from build123d import *

# Parameters (mm, degrees)
SZKIC1_R                         = 75
DODANIE_WYCI_GNI_CIE1_DEPTH      = 70
SKORUPA1_T                       = -2.5
SZKIC3_W                         = 13
SZKIC3_H                         = 21
WYTNIJ_WYCI_GNI_CIE1_DEPTH       = 60
SZKIC4_W                         = 9
SZKIC4_H                         = 11
WYTNIJ_WYCI_GNI_CIE2_DEPTH       = 60
DODANIE_WYCI_GNI_CIE2_REACH      = 192.066
DODANIE_WYCI_GNI_CIE2_END_RADIUS = 75
SZKIC7_W                         = 60
SZKIC7_H                         = 35
SZKIC8_W                         = 45.5
SZKIC8_H                         = 26.5
WYTNIJ_WYCI_GNI_CIE4_DEPTH       = 30
ZAOKR_GLENIE1_R                  = 5
WYTNIJ_WYCI_GNI_CIE5_DEPTH       = 14
SZKIC10_R                        = 1.5
WYTNIJ_WYCI_GNI_CIE6_DEPTH       = 10
SZYK_KO_OWY1_COUNT               = 4
PRZECI_CIE1_START                = -75.0000001
PRZECI_CIE1_OUTLINE_W            = 152
PRZECI_CIE1_OUTLINE_H            = 70
PRZECI_CIE1_OUTLINE_W_2          = 13
PRZECI_CIE1_OUTLINE_H_2          = 21
PRZECI_CIE1_OUTLINE_W_3          = 9
PRZECI_CIE1_OUTLINE_H_3          = 11
PRZECI_CIE1_DEPTH                = 75.0000001
SZKIC11_W                        = 10
SZKIC11_H                        = 10
SZKIC11_R                        = 2.5
DODANIE_WYCI_GNI_CIE3_DEPTH      = 4


# Read off the part's stored shape, not the designer's step: Przecięcie1
with BuildPart() as part:
    # Szkic1 → Dodanie-wyciągnięcie1 (new body)
    with BuildSketch(Plane.XY):
        Circle(SZKIC1_R)
    extrude(amount=DODANIE_WYCI_GNI_CIE1_DEPTH)

    # Skorupa1
    skorupa1_openings = [part.faces().sort_by_distance(p)[0] for p in [
        (0, 0, 70),
    ]]
    offset(amount=SKORUPA1_T, openings=skorupa1_openings, kind=Kind.INTERSECTION)

    # Szkic3 → Wytnij-wyciągnięcie1 (cut)
    with BuildSketch(Plane(origin=(0, -75, 0), x_dir=(-1, 0, 0), z_dir=(0, -1, 0))):
        with Locations((0, -35)):
            Rectangle(SZKIC3_W, SZKIC3_H)
    extrude(amount=-WYTNIJ_WYCI_GNI_CIE1_DEPTH, mode=Mode.SUBTRACT)

    # Szkic4 → Wytnij-wyciągnięcie2 (cut)
    with BuildSketch(Plane(origin=(0, -75, 0), x_dir=(-1, 0, 0), z_dir=(0, -1, 0))):
        with Locations((0, -14)):
            Rectangle(SZKIC4_W, SZKIC4_H)
    extrude(amount=-WYTNIJ_WYCI_GNI_CIE2_DEPTH, mode=Mode.SUBTRACT)

    # Dodanie-wyciągnięcie2: up to this cylinder (the profile starts outside it)
    dodanie_wyci_gni_cie2_end = Plane(origin=(0, 0, 35.532003), z_dir=(0, 0, -1)) * Cylinder(DODANIE_WYCI_GNI_CIE2_END_RADIUS, 535.132, mode=Mode.PRIVATE)
    # Szkic7 → Dodanie-wyciągnięcie2 (add, up to the surface)
    with BuildSketch(Plane(origin=(0, 85, 0), x_dir=(-1, 0, 0), z_dir=(0, -1, 0)), mode=Mode.PRIVATE) as dodanie_wyci_gni_cie2_sk1:
        with Locations((0, -35.532003496)):
            Rectangle(SZKIC7_W, SZKIC7_H)
    dodanie_wyci_gni_cie2_tool1 = extrude(dodanie_wyci_gni_cie2_sk1.sketch, amount=DODANIE_WYCI_GNI_CIE2_REACH, mode=Mode.PRIVATE) - dodanie_wyci_gni_cie2_end
    add(dodanie_wyci_gni_cie2_tool1.solids().sort_by_distance((0, 85, 35.532003))[0])

    # Szkic8 → Wytnij-wyciągnięcie4 (cut)
    with BuildSketch(Plane(origin=(0, 85, 0), x_dir=(1, 0, 0), z_dir=(0, 1, 0))):
        with Locations((0, -35.532003496)):
            Rectangle(SZKIC8_W, SZKIC8_H)
    extrude(amount=-WYTNIJ_WYCI_GNI_CIE4_DEPTH, mode=Mode.SUBTRACT)

    # Zaokrąglenie1
    zaokr_glenie1_edges = [part.edges().sort_by_distance(p)[0] for p in [
        (-30, 76.869317712, 18.032003496),
        (-30, 76.869317712, 53.032003496),
        (30, 76.869317712, 18.032003496),
        (30, 76.869317712, 53.032003496),
    ]]
    fillet(zaokr_glenie1_edges, radius=ZAOKR_GLENIE1_R)

    # Szkic9 → Wytnij-wyciągnięcie5 (cut)
    with BuildSketch(Plane(origin=(75, 0, 0), x_dir=(0, 0, -1), z_dir=(1, 0, 0))):
        with BuildLine():
            Line((-55, -12.979686846), (-55, 12.020313154))
            ThreePointArc((-55, 12.020313154), (-50, 17.020313154), (-45, 12.020313154))
            Line((-45, 12.020313154), (-45, -12.979686846))
            ThreePointArc((-45, -12.979686846), (-50, -17.979686846), (-55, -12.979686846))
        make_face()
    extrude(amount=-WYTNIJ_WYCI_GNI_CIE5_DEPTH, mode=Mode.SUBTRACT)

    # Szkic10 → Wytnij-wyciągnięcie6 (cut)
    with BuildSketch(Plane(origin=(53.033008589, 53.033008589, 0), x_dir=(0, 0, -1), z_dir=(0.7071067811865512, 0.7071067811865438, 0))):
        with Locations(Location((-66, 0, 0), (0, 0, 90))):
            Circle(SZKIC10_R)
    wytnij_wyci_gni_cie6 = extrude(amount=-WYTNIJ_WYCI_GNI_CIE6_DEPTH, mode=Mode.SUBTRACT)

    # Szyk kołowy1: Wytnij-wyciągnięcie6 ×4 about axis
    szyk_ko_owy1_axis = Axis((0, 0, 70), (0, 0, -1))
    for i in range(1, SZYK_KO_OWY1_COUNT):
        add(wytnij_wyci_gni_cie6.rotate(szyk_ko_owy1_axis, i * 360 / SZYK_KO_OWY1_COUNT), mode=Mode.SUBTRACT)

    # Przecięcie1 outline → Przecięcie1 (cut)
    with BuildSketch(Plane(origin=(0, 0, 0), x_dir=(1, 0, 0), z_dir=(0, 1, 0)).offset(PRZECI_CIE1_START)):
        with Locations((0, -35)):
            Rectangle(PRZECI_CIE1_OUTLINE_W, PRZECI_CIE1_OUTLINE_H)
        with Locations((0, -35)):
            Rectangle(PRZECI_CIE1_OUTLINE_W_2, PRZECI_CIE1_OUTLINE_H_2, mode=Mode.SUBTRACT)
        with Locations((0, -14)):
            Rectangle(PRZECI_CIE1_OUTLINE_W_3, PRZECI_CIE1_OUTLINE_H_3, mode=Mode.SUBTRACT)
    extrude(amount=PRZECI_CIE1_DEPTH, mode=Mode.SUBTRACT)

    # Szkic11 → Dodanie-wyciągnięcie3 (add)
    # profile 1 of 2: a face of its own
    with BuildSketch(Plane(origin=(0, 0, 0), x_dir=(-1, 0, 0), z_dir=(0, -1, 0))):
        with Locations((47.5, -7.5)):
            Rectangle(SZKIC11_W, SZKIC11_H)
        with Locations(Location((47.5, -8.5, 0), (0, 0, 90))):
            Circle(SZKIC11_R, mode=Mode.SUBTRACT)
    # profile 2 of 2: a face of its own
    with BuildSketch(Plane(origin=(0, 0, 0), x_dir=(-1, 0, 0), z_dir=(0, -1, 0))):
        with Locations((-47.5, -7.5)):
            Rectangle(SZKIC11_W, SZKIC11_H)
        with Locations(Location((-47.5, -8.5, 0), (0, 0, 90))):
            Circle(SZKIC11_R, mode=Mode.SUBTRACT)
    extrude(amount=-DODANIE_WYCI_GNI_CIE3_DEPTH)


solid = part.part
The listing builds one solid part. Answer for the finished solid, in the listing's coordinates (mm). A direction names the side the tool comes from. Coordinates: 2 decimals unless noted, no trailing zeros. Write each loop counter-clockwise with the first axis right and the second up, starting at its lowest first coordinate (ties: lowest second). Pieces come first, ordered by that corner, then holes. Notation, with made-up numbers: (65.25, 23) -> (108.25, 23) arc R9 cw to (108.25, 27) -> close; hole circle Ø1 at (9, -34.5). An arc over 180 degrees is marked (long way). One line per question, with ' | ' between items.
1. Straight lines are drawn through the part: line 1 (X direction, y = 2.45, z = 8.5); line 2 (X direction, y = 2, z = 8); line 3 (Z direction, x = 16.5, y = 63.5). For each, find the intervals that lie inside material, in ascending order.
Verdict:
line 1: x = -74.96 to -72.46, -52.5 to -50, -45 to -42.5, 42.5 to 45, 50 to 52.5, 72.46 to 74.96 | line 2: x = -74.97 to -72.47, -52.5 to -49.95, -45.05 to -42.5, 42.5 to 45.05, 49.95 to 52.5, 72.47 to 74.97 | line 3: z = 0 to 2.5
2. For a pull along Y with two mould halves and no side action, classify faces 4 (the flat face through (-47, 4, 5)), 5 (the flat face through (0, 85, 51)), 6 (the flat face through (0, 79, 48.782)) as released by +Y, released by -Y, zero draft, split by the parting line, or undercut.
Verdict:
face 4: undercut | face 5: released by +Y | face 6: zero draft
3. Section C-C (z = 8.5) is taken. Determine the outline of the cut face in (x, y), and give its area (3 significant figures).
Verdict:
outline: (-75, 0) -> (-72.5, 0) arc R72.5 cw to (72.5, 0) -> (75, 0) arc R75 ccw to start; (-52.5, 0) -> (-50, 0) -> (-50, 4) -> (-52.5, 4) -> close; (-45, 0) -> (-42.5, 0) -> (-42.5, 4) -> (-45, 4) -> close; (42.5, 0) -> (45, 0) -> (45, 4) -> (42.5, 4) -> close; (50, 0) -> (52.5, 0) -> (52.5, 4) -> (50, 4) -> close | area: 619 mm^2
4. Section D-D (x = 0) is taken. Determine the outline of the cut face in (y, z).
Verdict:
outline: (0, 0) -> (75, 0) -> (75, 18.03) -> (85, 18.03) -> (85, 22.28) -> (72.5, 22.28) -> (72.5, 2.5) -> (0, 2.5) -> close; (72.5, 48.78) -> (85, 48.78) -> (85, 53.03) -> (75, 53.03) -> (75, 70) -> (72.5, 70) -> close
5. Given pin 1 Ø4.5 at (x, y) = (-11.5, 78) entering from +Z; pin 2 Ø4.5 at (y, z) = (2, 5.5) entering from +X; pin 3 Ø12 at (x, z) = (55, 57.5) entering from -Y; pin 4 Ø4 at (y, z) = (67.5, 15.5) entering from -X, each flat-ended and moving along its own axis, determine where each tip first touches the part or whether it passes through.
Verdict:
pin 1: stops at z = 53.03 | pin 2: stops at x = 75 | pin 3: stops at y = 39.18 | pin 4: stops at x = -36.53
6. Section B-B (y = 77.5) is taken. Determine the outline of the cut face in (x, z), and give its area (3 significant figures).
Verdict:
outline: (-30, 23.03) arc R5 ccw to (-25, 18.03) -> (25, 18.03) arc R5 ccw to (30, 23.03) -> (30, 48.03) arc R5 ccw to (25, 53.03) -> (-25, 53.03) arc R5 ccw to (-30, 48.03) -> close; hole (-22.75, 22.28) -> (22.75, 22.28) -> (22.75, 48.78) -> (-22.75, 48.78) -> close | area: 873 mm^2
7. Section A-A (z = 25) is taken. Determine the outline of the cut face in (x, y).
Verdict:
outline: (-75, 0) -> (-72.5, 0) arc R72.5 cw to (-22.75, 68.84) -> (-22.75, 85) -> (-30, 85) -> (-30, 68.74) arc R75 ccw to start; (22.75, 68.84) arc R72.5 cw to (72.5, 0) -> (75, 0) arc R75 ccw to (30, 68.74) -> (30, 85) -> (22.75, 85) -> close
8. Which of the six approach directions +Z, -Z, +X, -X, +Y, -Y give full straight-line access (tool end or side, diameter ignored) to faces 1 (the flat face through (-22.75, 77, 36)), 2 (the flat face through (73, 6, 55)), 3 (the flat face through (42.5, 2, 8))?
Verdict:
face 1: +Y, -Y | face 2: +X, -Y | face 3: +Z, -Y
